Verification items for the finished model (mm, model axes). Face numbers are marked on the shaded views. A direction names the side the tool comes from. Give positions to 0.01 mm unless a question says otherwise; leave off trailing zeros. Loops run counter-clockwise (first coordinate to the right, second up) from the corner with the lowest first, then second, coordinate; pieces in that order, holes last. Notation, with made-up numbers: M 26,88 L 33,88 A34 cw 33,127 Z; hole C 75,59 d1. An arc over 180 degrees is marked long. Use a Markdown table: item, result.
from build123d import *

# Parameters (mm, degrees)
SKETCH_1_R      = 6.5
EXTRUDE_1_DEPTH = 125
SKETCH_2_R      = 4.9
EXTRUDE_2_DEPTH = 21
EXTRUDE_START   = 21
SKETCH_3_R      = 4.9
EXTRUDE_3_DEPTH = 21


with BuildPart() as part:
    # 草图1 → 凸台-拉伸1 (new body)
    with BuildSketch(Plane.XY):
        Circle(SKETCH_1_R)
    extrude(amount=EXTRUDE_1_DEPTH)

    # 草图2 → 凸台-拉伸2 (add)
    with BuildSketch(Plane.XY.offset(125)):
        with Locations(Location((0, 0, 0), (0, 0, 180))):
            Circle(SKETCH_2_R)
    extrude(amount=EXTRUDE_2_DEPTH)

    # 草图3 → 凸台-拉伸3 (add)
    with BuildSketch(Plane(origin=(0, 0, 0), x_dir=(-1, 0, 0), z_dir=(0, 0, -1)).offset(EXTRUDE_START)):
        Circle(SKETCH_3_R)
    extrude(amount=-EXTRUDE_3_DEPTH)


solid = part.part
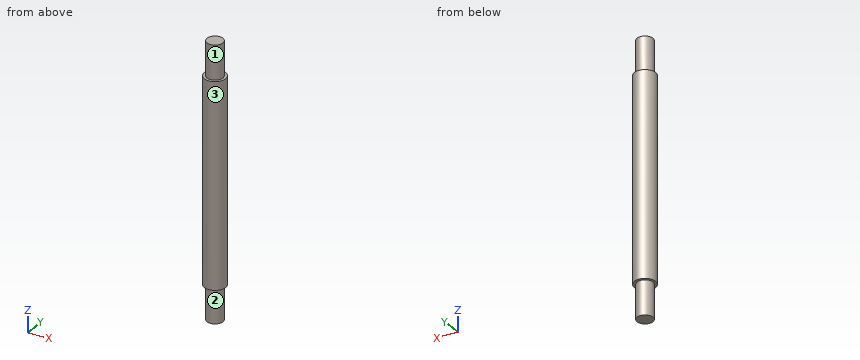
(1) Set-up check for the marked faces 1, 2 and 3: record each of +Z, -Z, +X, -X, +Y, -Y from which the full face is reachable in a straight line by a thin tool's end or side.
Results below:
| item | result |
|---|---|
| face 1 | +Z |
| face 2 | -Z |
| face 3 | +Z, -Z |
(2) Material ranges on line 1 (Z direction, x = 0.5, y = 5); line 2 (X direction, y = -0.5, z = 17.5), recorded low to high.
Results below:
| item | result |
|---|---|
| line 1 | 0 to 125 |
| line 2 | -6.48 to 6.48 |
(3) Cross-section at C-C on z = -2.5. Record the cut outline in (x, y), then the cut area to 3 significant figures.
Results below:
| item | result |
|---|---|
| outline | C 0,0 d9.8 |
| area | 75.4 mm^2 |
(4) Cross-section at D-D on z = 90.5. Record the cut outline in (x, y), then the cut area to 3 significant figures.
Results below:
| item | result |
|---|---|
| outline | C 0,0 d13 |
| area | 133 mm^2 |
(5) Cross-section at A-A on y = 0. Record the cut outline in (x, z).
Results below:
| item | result |
|---|---|
| outline | M -6.5,0 L -4.9,0 L -4.9,-21 L 4.9,-21 L 4.9,0 L 6.5,0 L 6.5,125 L 4.9,125 L 4.9,146 L -4.9,146 L -4.9,125 L -6.5,125 Z |
(6) Gauge pin test, flat ends, axial feed: P1, Ø3, axis at y = -4, z = 65.5, coming from the +X side; P2, Ø5, axis at x = -5, z = 50.5, coming from the -Y side; P3, Ø4, axis at y = -5, z = 99.5, coming from the +X side. Record the tip position at first contact, or that the pin passes through.
Results below:
| item | result |
|---|---|
| P1 | x = 6 |
| P2 | y = -6 |
| P3 | x = 5.77 |
